Read the model definition and answer for the solid it produces. Units are mm, in the model's axes. Face numbers are marked on the shaded views. Coordinates: 2 decimals unless noted, no trailing zeros. Order: outer loops, then holes, each group sorted by start corner. A loop starts at its lowest first (then second) coordinate and runs counter-clockwise, first axis right, second up. Notation, with made-up numbers: (54, -16) -> (106, -16) arc R24 ccw to (106, 9) -> close; hole circle Ø4 at (75.25, -15.75). An arc over 180 degrees is marked (long way). Use CSV: the item, a comma, the result in double quotes.
```python
from build123d import *

# Parameters (mm, degrees)
BOSS_EXTRUDE1_DEPTH = 78
SKETCH2_W           = 1.5
SKETCH2_H           = 75
BOSS_EXTRUDE2_DEPTH = 10
CUT_EXTRUDE1_REACH  = 119.339
SKETCH3_R           = 2.625
SKETCH4_W           = 78
SKETCH4_H           = 5
CUT_EXTRUDE2_DEPTH  = 118.338622692


with BuildPart() as part:
    # Sketch1 → Boss-Extrude1 (new body)
    with BuildSketch(Plane(origin=(0, 0, 0), x_dir=(0, 0, -1), z_dir=(1, 0, 0))):
        Polygon((0, 0), (0, 56.74), (56.74, 0), (51.08, 0), (4, 47.08), (4, 0), align=None)
    extrude(amount=BOSS_EXTRUDE1_DEPTH)

    # Sketch2 → Boss-Extrude2 (add)
    with BuildSketch(Plane(origin=(0, 28.37, -28.37), x_dir=(1, 0, 0), z_dir=(0, 0.7071067811865482, -0.7071067811865468))):
        with Locations((77.25, 2.621238765)):
            Rectangle(SKETCH2_W, SKETCH2_H)
    extrude(amount=BOSS_EXTRUDE2_DEPTH)

    # Sketch3 → Cut-Extrude1 (cut, up to next)
    with BuildSketch(Plane.XY, mode=Mode.PRIVATE) as cut_extrude1_sk1:
        with Locations((66, 25.86)):
            Circle(SKETCH3_R)
    cut_extrude1_tool1 = extrude(cut_extrude1_sk1.sketch, amount=-CUT_EXTRUDE1_REACH, mode=Mode.PRIVATE) & part.part
    # Sketch3 → Cut-Extrude1 (cut, up to next)
    with BuildSketch(Plane.XY, mode=Mode.PRIVATE) as cut_extrude1_sk2:
        with Locations((46, 25.86)):
            Circle(SKETCH3_R)
    cut_extrude1_tool2 = extrude(cut_extrude1_sk2.sketch, amount=-CUT_EXTRUDE1_REACH, mode=Mode.PRIVATE) & part.part
    add(cut_extrude1_tool1.solids().sort_by_distance((66, 25.86, 0))[0], mode=Mode.SUBTRACT)
    add(cut_extrude1_tool2.solids().sort_by_distance((46, 25.86, 0))[0], mode=Mode.SUBTRACT)

    # Sketch4 → Cut-Extrude2 (cut, through all)
    with BuildSketch(Plane.XY):
        with Locations((39, 2.5)):
            Rectangle(SKETCH4_W, SKETCH4_H)
    extrude(amount=-CUT_EXTRUDE2_DEPTH, mode=Mode.SUBTRACT)


solid = part.part
```
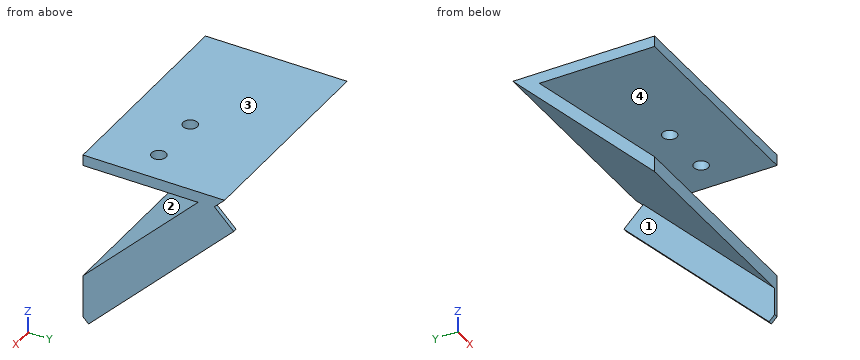
Item 1: Find section A-A, the plane y = 25.86. Give the vertices of the cut face in (x, z) (3 decimals).
Return value:
outline,"(0, -30.88) -> (76.5, -30.88) -> (76.5, -45.022) -> (78, -45.022) -> (78, -25.22) -> (0, -25.22) -> close; (0, -4) -> (43.375, -4) -> (43.375, 0) -> (0, 0) -> close; (48.625, -4) -> (63.375, -4) -> (63.375, 0) -> (48.625, 0) -> close; (68.625, -4) -> (78, -4) -> (78, 0) -> (68.625, 0) -> close"
Item 2: Each of these flat-tipped pins is pushed along its axis until it touches: P1, Ø2, axis at x = 14.5, z = -8.5, coming from the -Y side; P2, Ø4.5, axis at x = 46, y = 25.86, coming from the -Z side; P3, Ø10, axis at x = 33, z = -10.5, coming from the -Y side. Where does it stop, or does it pass through?
Return value:
P1,"stops at y = 41.58"
P2,"stops at z = -33.13"
P3,"stops at y = 35.58"
Item 3: Straight lines are drawn through the part: line 1 along X through (y, z) = (25, -3); line 2 along Z through (x, y) = (21, 38); line 3 along Z through (x, y) = (25, 24.5). For each, find the intervals that lie inside material, in ascending order.
Return value:
line 1,"x = 0 to 43.52, 48.48 to 63.52, 68.48 to 78"
line 2,"z = -18.74 to -13.08, -4 to 0"
line 3,"z = -32.24 to -26.58, -4 to 0"
Item 4: Find section D-D, the plane z = -47.5. Give the vertices of the cut face in (x, y), then the cut area to 3 significant figures.
Return value:
outline,"(0, 5) -> (78, 5) -> (78, 23.38) -> (76.5, 23.38) -> (76.5, 9.24) -> (0, 9.24) -> close"
area,"352 mm^2"
Item 5: The mould has two halves that part along Z. Classify the marked faces 1, 2, 3 and 4: +Z half, -Z half, draft (parallel to the pull), parting line (faces both ways), or undercut.
Return value:
face 1,"draft"
face 2,"undercut"
face 3,"+Z half"
face 4,"undercut"
Item 6: Find section C-C, the plane y = 18. Give the vertices of the cut face in (x, z), then the cut area to 3 significant figures.
Return value:
outline,"(0, -38.74) -> (76.5, -38.74) -> (76.5, -52.88) -> (78, -52.88) -> (78, -33.08) -> (0, -33.08) -> close; (0, -4) -> (78, -4) -> (78, 0) -> (0, 0) -> close"
area,"775 mm^2"
Item 7: Find section B-B, the plane x = 66.5. Give the vertices of the cut face in (y, z), then the cut area to 3 significant figures.
Return value:
outline,"(5, -51.74) -> (56.74, 0) -> (28.44, 0) -> (28.44, -4) -> (47.08, -4) -> (5, -46.08) -> close; (5, -4) -> (23.28, -4) -> (23.28, 0) -> (5, 0) -> close"
area,"433 mm^2"
